Autodesk Fusion 360 part; units mm, degrees
sketch "Sketch1" plane through (0, 0, 0) normal (0, 1, 0) x (1, 0, 0)
  circle A0 centre (0, 0) radius 14
  circle A1 centre (0, 0) radius 17 construction
  circle A2 centre (0, 0) radius 26
  arc A3 (14.7224, -8.5) -> (17, 0) centre (0, 0) ccw
  line L0 (0, 0) -> (14.7224, -8.5) construction
  line L1 (0, 0) -> (17, 0) construction
  circle A4 centre (14.7224, -8.5) radius 0.9
  circle A5 centre (0, 17) radius 0.9
  circle A6 centre (-14.7224, -8.5) radius 0.9
  dimension "d1" = 28
  dimension "d2" = 34
  dimension "d3" = 52
  dimension "d4" = 30
  dimension "d5" = 1.8
  dimension "d7" = 360
extrude "Extrude1" add sketch "Sketch1" along normal blind 1
The listing builds one solid part. Answer for the finished solid, in the listing's coordinates (mm). Give positions to 0.01 mm unless a question says otherwise; leave off trailing zeros. Order: outer loops, then holes, each group sorted by start corner. A loop starts at its lowest first (then second) coordinate and runs counter-clockwise, first axis right, second up.
Item 1: For a pull along X with two mould halves and no side action, classify faces 1 (the face through (-20.633, 0.493, -15.821)), 2 (the face through (-14.24, 0.49, 9.26)), 3 (the face through (11, 0, 11)) as pulls with the +X half, pulls with the -X half, needs draft (parallel to the pull), parting line crosses it, or undercut.
From the geometry:
face 1: parting line crosses it
face 2: undercut
face 3: needs draft
Item 2: Find the intervals of material crossed by probe 1 along X at (y, z) = (0.4, 0); probe 2 along X at (y, z) = (0.7, 8.5); probe 3 along X at (y, z) = (0.45, -17), in increasing order.
From the geometry:
probe 1: x = -26 to -14, 14 to 26
probe 2: x = -24.57 to -15.62, -13.82 to -11.12, 11.12 to 13.82, 15.62 to 24.57
probe 3: x = -19.67 to -0.9, 0.9 to 19.67
Item 3: The part is cut by section A-A, the plane x = 0. Give the vertices of the cut face in (y, z).
From the geometry:
outline: (0, -26) - (1, -26) - (1, -17.9) - (0, -17.9) - close; (0, -16.1) - (1, -16.1) - (1, -14) - (0, -14) - close; (0, 14) - (1, 14) - (1, 26) - (0, 26) - close
Item 4: The part is cut by section C-C, the plane y = 0.2. Give the vertices of the cut face in (x, z), and give its area (3 significant figures).
From the geometry:
outline: circle Ø52 at (0, 0); hole circle Ø1.8 at (-14.72, 8.5); hole circle Ø28 at (0, 0); hole circle Ø1.8 at (0, -17); hole circle Ø1.8 at (14.72, 8.5)
area: 1,500 mm2
Item 5: The part is cut by section D-D, the plane x = -15. Give the vertices of the cut face in (y, z).
From the geometry:
outline: (0, -21.24) - (1, -21.24) - (1, 7.64) - (0, 7.64) - close; (0, 9.36) - (1, 9.36) - (1, 21.24) - (0, 21.24) - close
Item 6: The part is cut by section B-B, the plane z = 0. Give the vertices of the cut face in (x, y), and give its area (3 significant figures).
From the geometry:
outline: (-26, 0) - (-14, 0) - (-14, 1) - (-26, 1) - close; (14, 0) - (26, 0) - (26, 1) - (14, 1) - close
area: 24.0 mm2
